from build123d import *

# Parameters (mm, degrees)
F0_W      = 10
F0_H      = 3
F0_W_2    = 7.1
F0_H_2    = 12.3
F1_DEPTH  = 10
F2_R      = 1.4483503842
F1_FACE_W = 21.323674424
F1_FACE_H = 10
F3_DEPTH  = 15.301
F4_R      = 4.99999
F5_F1_R   = 1
F5_F2_R   = 1
F5_F3_R   = 1
F5_F4_R   = 1
F5_F5_R   = 1
F5_F6_R   = 1
F5_F7_R   = 1
F5_F8_R   = 1
F5_F9_R   = 1
F5_F10_R  = 0.9999
F5_F11_R  = 1
F5_F12_R  = 1
F5_F13_R  = 1


# Not quite as in the source:
# - a fillet or chamfer is up to 0.001 mm smaller than in the source, because OpenCascade refuses the exact size


with BuildPart() as f1:
    # F0 (on Top) → F1 (new body)
    with BuildSketch(Plane.XY):
        with Locations((14.223674424, 13.8)):
            Rectangle(F0_W, F0_H)
        Polygon((-2.1, 12.3), (-2.1, 0), (-2.1, -2.1), (7.1, -2.1), (9.223674424, -2.1), (9.223674424, 12.3), (9.223674424, 15.3), (-2.1, 15.3), (-2.1, 14.4), (-2.0836676853, 12.3), align=None)
        with Locations((3.55, 6.15)):
            Rectangle(F0_W_2, F0_H_2, mode=Mode.SUBTRACT)
    extrude(amount=F1_DEPTH)

    # F2 (on Front) + F1_face (on face) → F3 (cut, through all)
    with BuildSketch(Plane.XZ):
        with Locations((14.2455906607, 4.9976706505)):
            Circle(F2_R)
    with BuildSketch(Plane(origin=(8.561837212, 15.3, 5), x_dir=(-1, 0, 0), z_dir=(0, 1, 0))):
        Rectangle(F1_FACE_W, F1_FACE_H)
    extrude(amount=-F3_DEPTH, dir=(0, -1, 0), mode=Mode.SUBTRACT)

    # F4 (radius 5 in the source; OpenCascade refuses exactly that, so slightly less here)
    f4_edges = [f1.edges().sort_by_distance(p)[0] for p in [
        (19.223674, 13.8, 10),
        (19.223674, 13.8, 0),
    ]]
    fillet(f4_edges, radius=F4_R)

    # F5: fillet of radius 1 on 18 edges, made by hand

    # F5_f1
    f5_f1_edges = [f1.edges().sort_by_distance(p)[0] for p in [
        (9.223674424, 5.1, 0),
    ]]
    fillet(f5_f1_edges, radius=F5_F1_R)

    # F5_f2
    f5_f2_edges = [f1.edges().sort_by_distance(p)[0] for p in [
        (-2.1, 5.1, 0),
    ]]
    fillet(f5_f2_edges, radius=F5_F2_R)

    # F5_f3
    f5_f3_edges = [f1.edges().sort_by_distance(p)[0] for p in [
        (9.223674424, 5.1, 10),
    ]]
    fillet(f5_f3_edges, radius=F5_F3_R)

    # F5_f4
    f5_f4_edges = [f1.edges().sort_by_distance(p)[0] for p in [
        (-2.1, 5.1, 10),
    ]]
    fillet(f5_f4_edges, radius=F5_F4_R)

    # F5_f5
    f5_f5_edges = [f1.edges().sort_by_distance(p)[0] for p in [
        (0, 6.15, 0),
    ]]
    fillet(f5_f5_edges, radius=F5_F5_R)

    # F5_f6
    f5_f6_edges = [f1.edges().sort_by_distance(p)[0] for p in [
        (7.1, 6.15, 0),
    ]]
    fillet(f5_f6_edges, radius=F5_F6_R)

    # F5_f7
    f5_f7_edges = [f1.edges().sort_by_distance(p)[0] for p in [
        (0, 6.15, 10),
    ]]
    fillet(f5_f7_edges, radius=F5_F7_R)

    # F5_f8
    f5_f8_edges = [f1.edges().sort_by_distance(p)[0] for p in [
        (7.1, 6.15, 10),
    ]]
    fillet(f5_f8_edges, radius=F5_F8_R)

    # F5_f9
    f5_f9_edges = [f1.edges().sort_by_distance(p)[0] for p in [
        (3.561837212, -2.1, 0),
    ]]
    fillet(f5_f9_edges, radius=F5_F9_R)

    # F5_f10 (radius 1 in the source; OpenCascade refuses exactly that, so slightly less here)
    f5_f10_edges = [f1.edges().sort_by_distance(p)[0] for p in [
        (3.55, 12.3, 0),
    ]]
    fillet(f5_f10_edges, radius=F5_F10_R)

    # F5_f11
    f5_f11_edges = [f1.edges().sort_by_distance(p)[0] for p in [
        (3.55, 0, 0),
    ]]
    fillet(f5_f11_edges, radius=F5_F11_R)

    # F5_f12
    f5_f12_edges = [f1.edges().sort_by_distance(p)[0] for p in [
        (3.55, 12.3, 10),
    ]]
    fillet(f5_f12_edges, radius=F5_F12_R)

    # F5_f13
    f5_f13_edges = [f1.edges().sort_by_distance(p)[0] for p in [
        (3.55, 0, 10),
    ]]
    fillet(f5_f13_edges, radius=F5_F13_R)


solid = f1.part
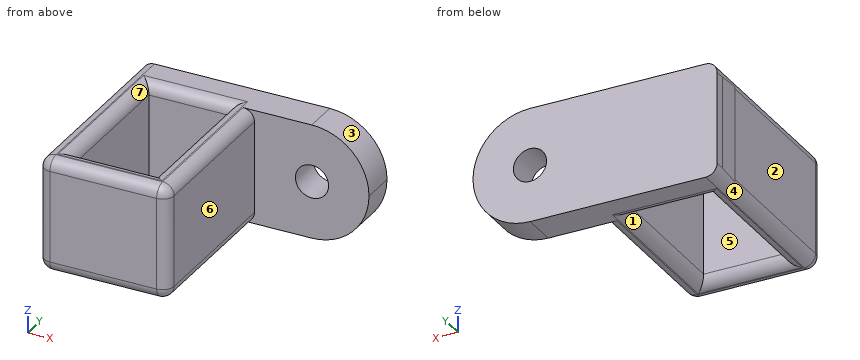
Geometry check sheet. Reference: the model listing, model coordinates, mm. Face numbers are marked on the shaded views. A direction names the side the tool comes from. Coordinates: 2 decimals unless noted, no trailing zeros. Order: outer loops, then holes, each group sorted by start corner. A loop starts at its lowest first (then second) coordinate and runs counter-clockwise, first axis right, second up. Notation, with made-up numbers: (-0.5, 44.25) - (35.5, 44.25) arc R26 cw to (35.5, 71.25) - close; hole circle Ø11 at (27, 14.25). An arc over 180 degrees is marked (long way). Answer in a Markdown table with one row per item. Add a question column.
1) Cross-section at A-A, the plane x = 6. Record the cut outline in (y, z).
2) Set-up check for the marked faces 4, 5, 6 and 7: record each of +Z, -Z, +X, -X, +Y, -Y from which the full face is reachable in a straight line by a thin tool's end or side.
3) Material ranges on line 1 along X through (y, z) = (4.25, 1.5); line 2 along Y through (x, z) = (6.25, 4.5); line 3 along Y through (x, z) = (17.5, 7.25), recorded low to high. Write a range as [from, to].
4) Cross-section at C-C, the plane z = 4.5. State how many separate pieces and enclosed holes the cut face has, then the cut area to 3 significant figures.
5) Cross-section at B-B, the plane y = 7.75. Record the cut outline in (x, z).
6) Gauge pin test, flat ends, axial feed: P1, Ø6, axis at y = 6.5, z = 1.5, coming from the +X side; P2, Ø1.7, axis at x = 14.25, z = 5, coming from the -Y side. Record the tip position at first contact, or that the pin passes through.
7) Release check for a two-part mould opening along X. For the marked faces 1, 2 and 3 record: +X half, -X half, draft (parallel to the pull), parting line (faces both ways), or undercut.
Check result:
| question | item | result |
|---|---|---|
| 1 | outline | (-2.1, 1) arc R1 ccw to (-1.1, 0) - (-1, 0) arc R1 ccw to (0, 1) - (0, 9) arc R1 ccw to (-1, 10) - (-1.1, 10) arc R1 ccw to (-2.1, 9) - close; (12.3, 1) arc R1 ccw to (13.3, 0) - (15.3, 0) - (15.3, 10) - (13.3, 10) arc R1 ccw to (12.3, 9) - close |
| 2 | face 4 | -Z, -X, +Y, -Y |
| 2 | face 5 | +Z, -Z |
| 2 | face 6 | +Z, -Z, +X, -Y |
| 2 | face 7 | +Z |
| 3 | line 1 | x = [-2.1, 0], [7.1, 9.22] |
| 3 | line 2 | y = [-2.1, 0], [12.3, 15.3] |
| 3 | line 3 | y = [12.3, 15.3] |
| 4 | separate pieces | 2 |
| 4 | enclosed holes | 1 |
| 4 | area | 131 mm² |
| 5 | outline | (-2.1, 1) arc R1 ccw to (-1.1, 0) - (-1, 0) arc R1 ccw to (0, 1) - (0, 9) arc R1 ccw to (-1, 10) - (-1.1, 10) arc R1 ccw to (-2.1, 9) - close; (7.1, 1) arc R1 ccw to (8.1, 0) - (8.22, 0) arc R1 ccw to (9.22, 1) - (9.22, 9) arc R1 ccw to (8.22, 10) - (8.1, 10) arc R1 ccw to (7.1, 9) - close |
| 6 | P1 | stops at x = 9.22 |
| 6 | P2 | passes through |
| 7 | face 1 | undercut |
| 7 | face 2 | -X half |
| 7 | face 3 | +X half |
